Could you check a few things on this drawing? It's one solid part, dimensions in mm from its lowest x, y, z. A direction names the side the tool comes from. Round coordinates to 2 decimals unless told otherwise and drop trailing zeros. Write each loop counter-clockwise with the first axis right and the second up, starting at its lowest first coordinate (ties: lowest second). Pieces come first, ordered by that corner, then holes. Notation, with made-up numbers: (43, 10) -> (55, 10) arc R20 cw to (55, 47) -> close; hole circle Ø4 at (14.5, 27). An arc over 180 degrees is marked (long way). Answer in a Markdown table with one row per item.
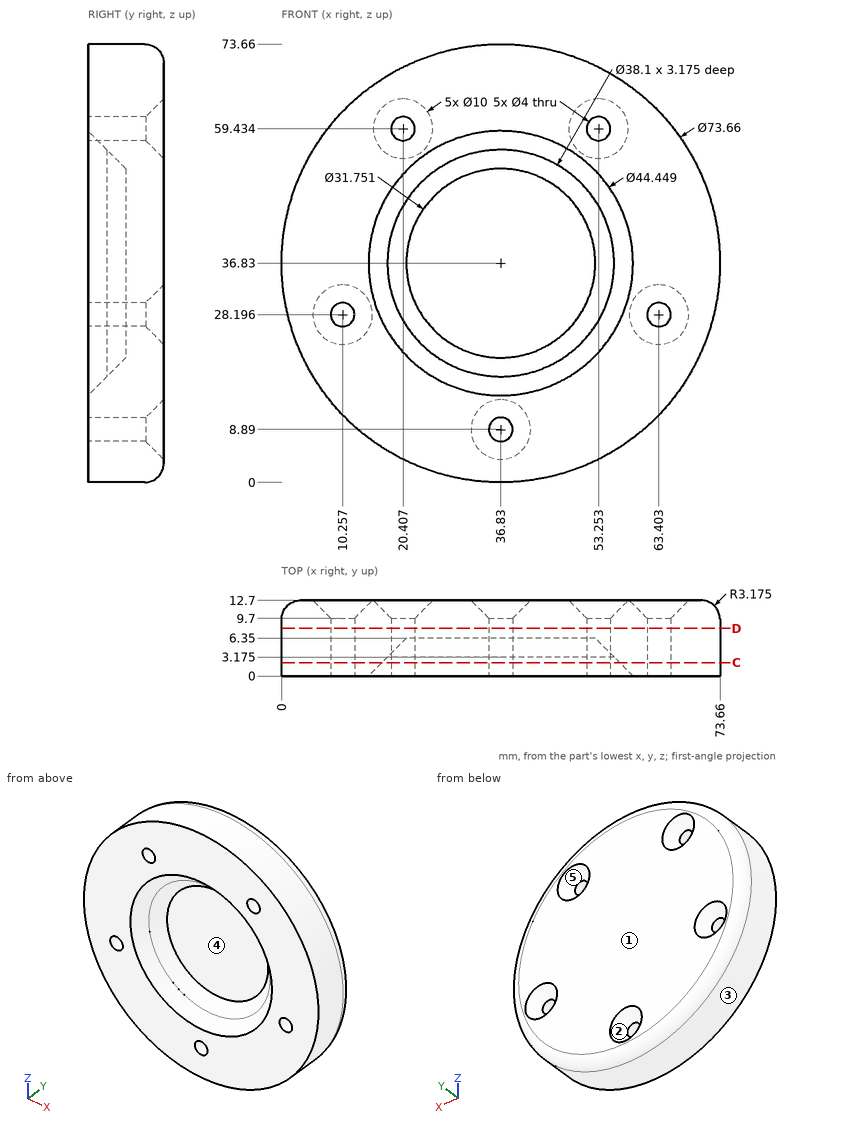
1) Please list where these lines run through material, in increasing order: line 1 (Z direction, x = 35.5, y = 4.5) (1 decimal); line 2 (X direction, y = 1.25, z = 60) (1 decimal); line 3 (Z direction, x = 64, y = 3.75) (1 decimal).
Findings:
| item | result |
|---|---|
| line 1 | z = 0 to 7.4, 10.4 to 19.2, 54.5 to 73.6 |
| line 2 | x = 8.2 to 18.5, 22.3 to 51.3, 55.2 to 65.5 |
| line 3 | z = 12 to 26.3, 30.1 to 61.7 |
2) Imagine slicing it at C-C, the plane y = 2.25. Count the separate pieces of the cut face and the enclosed holes in it.
Findings:
| item | result |
|---|---|
| separate pieces | 1 |
| enclosed holes | 6 |
3) Thinking about a two-plate mould opening in X: for the marked faces 1, 2 and 3, which applies, +X half, -X half, draft (parallel to the pull), parting line (faces both ways), or undercut?
Findings:
| item | result |
|---|---|
| face 1 | draft |
| face 2 | undercut |
| face 3 | parting line |
4) For pin 1 (6.5 mm diameter, centred on x = 36.83, z = 8.89, fed in from +Y); pin 2 (6 mm diameter, centred on x = 54.5, y = 10, fed in from -Z); pin 3 (10 mm diameter, centred on x = 47, z = 47, fed in from -Y); pin 4 (2 mm diameter, centred on x = 57, z = 16, fed in from -Y), each with a flat end and sliding along its axis, tell me the tip position at first contact or that it passes through.
Findings:
| item | result |
|---|---|
| pin 1 | stops at y = 10.95 |
| pin 2 | stops at z = 3.06 |
| pin 3 | stops at y = 2.84 |
| pin 4 | stops at y = 0 |
5) For the marked faces 4 and 5, which set-ups out of +Z, -Z, +X, -X, +Y, -Y let a thin tool reach every point of the face, with its end or its side?
Findings:
| item | result |
|---|---|
| face 4 | -Y |
| face 5 | +Y |
6) Imagine slicing it at D-D, the plane y = 8. Please give me the cut outline in (x, z).
Findings:
| item | result |
|---|---|
| outline | circle Ø73.66 at (36.83, 36.83); hole circle Ø4 at (10.26, 28.2); hole circle Ø4 at (20.41, 59.43); hole circle Ø4 at (36.83, 8.89); hole circle Ø4 at (53.25, 59.43); hole circle Ø4 at (63.4, 28.2) |
